Read the model definition and answer for the solid it produces. Units are mm, in the model's axes. Face numbers are marked on the shaded views. Give positions to 0.01 mm unless a question says otherwise; leave off trailing zeros. Order: outer loops, then holes, each group sorted by start corner. A loop starts at its lowest first (then second) coordinate and runs counter-clockwise, first axis right, second up.
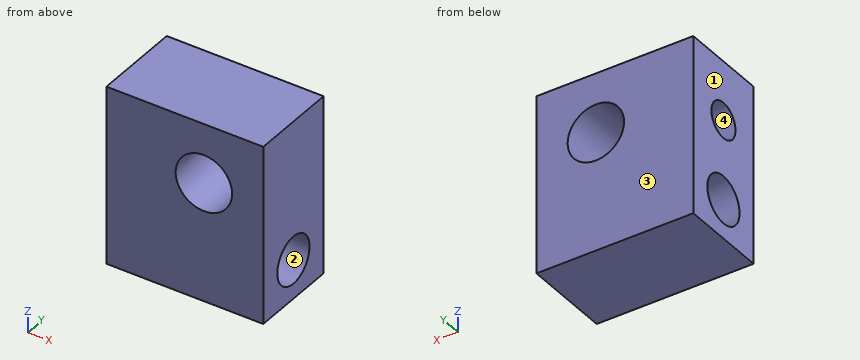
Autodesk Inventor part; units mm, degrees
ref_plane "YZ Plane" through (0, 0, 0) normal (1, 0, 0) x (0, 1, 0)
ref_plane "XZ Plane" through (0, 0, 0) normal (0, 1, 0) x (-1, 0, 0)
ref_plane "XY Plane" through (0, 0, 0) normal (0, 0, 1) x (1, 0, 0)
sketch "Sketch1" plane through (0, 0, 0) normal (0, 1, 0) x (-1, 0, 0)
  line L0 (0, 0) -> (26.4, 0)
  line L1 (26.4, 0) -> (26.4, -30)
  line L2 (26.4, -30) -> (0, -30)
  line L3 (0, -30) -> (0, 0)
  dimension "d0" = 26.4
  dimension "d1" = 30
extrude "Extrusion1" add sketch "Sketch1" along normal blind 15
sketch "Sketch2" plane through (0, 15, 0) normal (0, 1, 0) x (1, 0, 0)
  circle A0 centre (-10, 10) radius 4.75
  line L0 (0, 0) -> (0, 30)
  line L1 (-26.4, 0) -> (0, 0)
  dimension "d4" = 9.5
  dimension "d5" = 10
  dimension "d6" = 10
extrude "Extrusion2" cut sketch "Sketch2" against normal blind 15
sketch "Sketch3" plane through (-26.4, 0, -30) normal (-1, 0, 0) x (0, 0, 1)
  line L0 (24.75, 0) -> (15.25, 0)
  line L1 (15.25, 15) -> (24.75, 15)
  line L2 (24.75, 15) -> (24.75, 0)
  line L3 (15.25, 15) -> (15.25, 0)
  circle A0 centre (20, 7.5) radius 2
  point P0 (30, 0)
  dimension "d12" = 4
hole "Hole1" at (-26.4, 7.5, -10) direction (1, 0, 0) diameter 6 depth 8 tip angle 120
sketch "Sketch4" plane through (-26.4, 0, -30) normal (-1, 0, 0) x (0, 0, 1)
  line L0 (0, 0) -> (0, 15)
  circle A0 centre (6.5597, 7.5) radius 4
  point P0 (30, 0)
  dimension "d20" = 8
extrude "Extrusion3" cut sketch "Sketch4" against normal blind 32.75
thread "Thread1"
thread "Thread2"
properties part number "КВ33.000.109 - Каретка"
1) Given pin 1 (5 mm diameter, centred on x = -8.5, z = -8, fed in from -Y); pin 2 (5.5 mm diameter, centred on y = 7.5, z = -10, fed in from -X), each flat-ended and moving along its own axis, determine where each tip first touches the part or whether it passes through.
Final values:
pin 1: stops at y = 0
pin 2: stops at x = -18.26
2) For a pull along Y with two mould halves and no side action, classify the marked faces 1, 2, 3 and 4 as released by +Y, released by -Y, zero draft, split by the parting line, or undercut.
Final values:
face 1: zero draft
face 2: undercut
face 3: released by +Y
face 4: undercut
3) The part is cut by section C-C on x = -2. Determine the outline of the cut face in (y, z), and give its area (3 significant figures).
Final values:
outline: (0, -30) - (15, -30) - (15, 0) - (0, 0) - close; hole circle Ø8 at (7.5, -23.44)
area: 400 mm2
4) The part is cut by section B-B on z = -22. Determine the outline of the cut face in (x, y).
Final values:
outline: (-26.4, 0) - (0, 0) - (0, 3.77) - (-26.4, 3.77) - close; (-26.4, 11.23) - (0, 11.23) - (0, 15) - (-26.4, 15) - close
5) Consider L1, parallel to Z at x = -9.5, y = 4.75; L2, parallel to Y at x = -23.25, z = -22.5; L3, parallel to Z at x = -24.5, y = 8.5. Determine where each line is inside the solid, lowest interval first.
Final values:
L1: z = -30 to -26.35, -20.54 to -14.72, -5.28 to 0
L2: y = 0 to 3.61, 11.39 to 15
L3: z = -30 to -27.31, -19.57 to -12.83, -7.17 to 0
6) The part is cut by section D-D on x = -20.75. Determine the outline of the cut face in (y, z).
Final values:
outline: (0, -30) - (15, -30) - (15, 0) - (0, 0) - close; hole circle Ø8 at (7.5, -23.44); hole circle Ø6 at (7.5, -10)
7) The part is cut by section A-A on x = -8. Determine the outline of the cut face in (y, z), and give its area (3 significant figures).
Final values:
outline: (0, -30) - (15, -30) - (15, -14.31) - (0, -14.31) - close; (0, -5.69) - (15, -5.69) - (15, 0) - (0, 0) - close; hole circle Ø8 at (7.5, -23.44)
area: 270 mm2
